Read the model definition and answer for the solid it produces. Units are mm, in the model's axes. Face numbers are marked on the shaded views. A direction names the side the tool comes from. Give positions to 0.01 mm unless a question says otherwise; leave off trailing zeros. Write each loop counter-clockwise with the first axis right and the second up, starting at its lowest first coordinate (ties: lowest second). Pieces come first, ordered by that corner, then holes. Notation, with made-up numbers: M 83.5,-4 L 106.5,-4 A3 ccw 106.5,0 Z; hole C 29,26.25 d6. An arc over 180 degrees is marked long. Put each result on its own line as item: value.
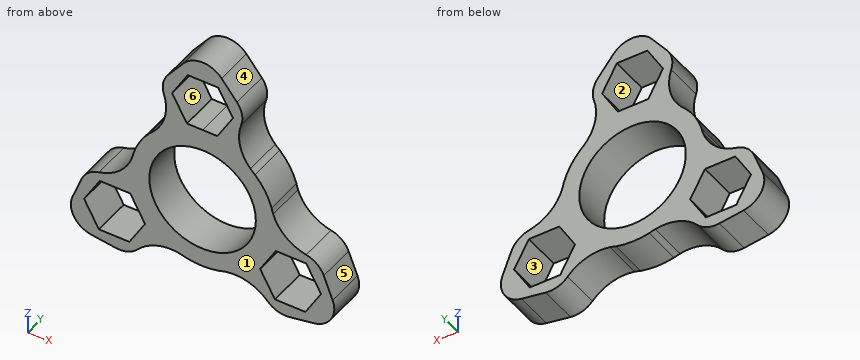
from build123d import *

# Parameters (mm, degrees)
F0_R     = 10.9
F1_DEPTH = 8
F2_R     = 5


with BuildPart() as f1:
    # F0 (on Front) → F1 (new body)
    with BuildSketch(Plane.XZ):
        with BuildLine():
            ThreePointArc((-4.6474292299, -13.9936443391), (-12.7697106566, -7.372595885), (-14.4425661041, 2.9720303942))
            ThreePointArc((-14.4425661041, 2.9720303942), (-17.9890829323, -1.7394577094), (-23.6744608764, -3.305465179))
            Line((-23.6744608764, -3.305465179), (-26.6141080798, -10.8626586404))
            ThreePointArc((-26.6141080798, -10.8626586404), (-26.2843656104, -15.1752855606), (-22.7143923751, -17.617164376))
            Line((-22.7143923751, -17.617164376), (-14.6998472546, -18.8499519504))
            ThreePointArc((-14.6998472546, -18.8499519504), (-10.5009560313, -14.7092739554), (-4.6474292299, -13.9936443391))
        make_face()
        Polygon((-21.2154018643, -15.7464514283), (-24.2445278885, -10.2962775292), (-21.039101849, -4.9478904915), (-14.8045497853, -5.0496773528), (-11.7754237611, -10.4998512519), (-14.9808498006, -15.8482382896), align=None, mode=Mode.SUBTRACT)
        with BuildLine():
            ThreePointArc((9.7951368743, 11.0216139449), (5.2395070905, 13.7828968575), (0, 14.7451917701))
            ThreePointArc((0, 14.7451917701), (-5.2395070905, 13.7828968575), (-9.7951368743, 11.0216139449))
            ThreePointArc((-9.7951368743, 11.0216139449), (-10.2405850834, 10.5580719376), (-10.7175072848, 10.1269797045))
            ThreePointArc((-10.7175072848, 10.1269797045), (-12.7697106566, 7.372595885), (-14.1289753301, 4.2181437217))
            ThreePointArc((-14.1289753301, 4.2181437217), (-14.2638510546, 3.5895708631), (-14.4425661041, 2.9720303942))
            ThreePointArc((-14.4425661041, 2.9720303942), (-12.7697106566, -7.372595885), (-4.6474292299, -13.9936443391))
            ThreePointArc((-4.6474292299, -13.9936443391), (-4.0232659712, -14.1476428006), (-3.4114680453, -14.3451234262))
            ThreePointArc((-3.4114680453, -14.3451234262), (0, -14.7451917701), (3.4114680453, -14.3451234262))
            ThreePointArc((3.4114680453, -14.3451234262), (4.0232659712, -14.1476428006), (4.6474292299, -13.9936443391))
            ThreePointArc((4.6474292299, -13.9936443391), (11.9571718138, -8.6282514191), (14.7451917701, 0))
            ThreePointArc((14.7451917701, 0), (14.6693402577, 1.4936990123), (14.4425661041, 2.9720303942))
            ThreePointArc((14.4425661041, 2.9720303942), (14.2638510546, 3.5895708631), (14.1289753301, 4.2181437217))
            ThreePointArc((14.1289753301, 4.2181437217), (12.7697106566, 7.372595885), (10.7175072848, 10.1269797045))
            ThreePointArc((10.7175072848, 10.1269797045), (10.2405850834, 10.5580719376), (9.7951368743, 11.0216139449))
        make_face()
        Circle(F0_R, mode=Mode.SUBTRACT)
        with BuildLine():
            ThreePointArc((23.6744608764, -3.305465179), (17.9890829323, -1.7394577094), (14.4425661041, 2.9720303942))
            ThreePointArc((14.4425661041, 2.9720303942), (14.6693402577, 1.4936990123), (14.7451917701, 0))
            ThreePointArc((14.7451917701, 0), (11.9571718138, -8.6282514191), (4.6474292299, -13.9936443391))
            ThreePointArc((4.6474292299, -13.9936443391), (10.5009560313, -14.7092739554), (14.6998472546, -18.8499519504))
            Line((14.6998472546, -18.8499519504), (22.7143923751, -17.617164376))
            ThreePointArc((22.7143923751, -17.617164376), (26.2843656104, -15.1752855606), (26.6141080798, -10.8626586404))
            Line((26.6141080798, -10.8626586404), (23.6744608764, -3.305465179))
        make_face()
        Polygon((24.2445278885, -10.4998512519), (21.039101849, -15.8482382896), (14.8045497853, -15.7464514283), (11.7754237611, -10.2962775292), (14.9808498006, -4.9478904915), (21.2154018643, -5.0496773528), align=None, mode=Mode.SUBTRACT)
        with BuildLine():
            ThreePointArc((-9.7951368743, 11.0216139449), (-5.2395070905, 13.7828968575), (0, 14.7451917701))
            ThreePointArc((0, 14.7451917701), (5.2395070905, 13.7828968575), (9.7951368743, 11.0216139449))
            ThreePointArc((9.7951368743, 11.0216139449), (7.488126901, 16.4487316648), (8.9746136218, 22.1554171294))
            Line((8.9746136218, 22.1554171294), (3.8997157047, 28.4798230164))
            ThreePointArc((3.8997157047, 28.4798230164), (0, 30.3505711213), (-3.8997157047, 28.4798230164))
            Line((-3.8997157047, 28.4798230164), (-8.9746136218, 22.1554171294))
            ThreePointArc((-8.9746136218, 22.1554171294), (-7.488126901, 16.4487316648), (-9.7951368743, 11.0216139449))
        make_face()
        Polygon((3.0291260242, 15.3459548821), (0, 15.3954091536), (-3.2054260395, 15.4477417434), (-6.2345520637, 20.8979156424), (-3.0291260242, 26.2463026801), (3.2054260395, 26.1445158188), (6.2345520637, 20.6943419198), align=None, mode=Mode.SUBTRACT)
    extrude(amount=F1_DEPTH)

    # F2
    f2_edges = [f1.edges().sort_by_distance(p)[0] for p in [
        (-23.674461, -4, -3.305465),
        (-14.699847, -4, -18.849952),
        (14.699847, -4, -18.849952),
        (23.674461, -4, -3.305465),
        (8.974614, -4, 22.155417),
        (-8.974614, -4, 22.155417),
    ]]
    fillet(f2_edges, radius=F2_R)


solid = f1.part
(1) Which of the six approach directions +Z, -Z, +X, -X, +Y, -Y give full straight-line access (tool end or side, diameter ignored) to the marked faces 5 and 6?
Result:
face 5: +Z, +X, +Y, -Y
face 6: +Y, -Y
(2) Section B-B on z = 0 is taken. Determine the outline of the cut face in (x, y).
Result:
outline: M -16.08,-8 L -10.9,-8 L -10.9,0 L -16.08,0 Z; M 10.9,-8 L 16.08,-8 L 16.08,0 L 10.9,0 Z
(3) Straight lines are drawn through the part: line 1 along Z through (x, y) = (-0.5, -7); line 2 along X through (y, z) = (-5.75, -15.5); line 3 along Z through (x, y) = (1, -0.5). For each, find the intervals that lie inside material, in ascending order. Write a range as from..to.
Result:
line 1: z = -14.74..-10.89, 10.89..15.4, 26.21..30.33
line 2: x = -26.08..-21.35, -14.77..-11.84, 11.84..14.67, 21.25..26.08
line 3: z = -14.71..-10.85, 10.85..15.38, 26.18..30.25
(4) Section C-C on y = -2.5 is taken. Give the number of separate pieces and of enclosed holes in the cut face, and give its area (3 significant figures).
Result:
separate pieces: 1
enclosed holes: 4
area: 663 mm²
(5) Section A-A on x = -19 is taken. Determine the outline of the cut face in (y, z), and give its area (3 significant figures).
Result:
outline: M -8,-18.19 L 0,-18.19 L 0,-15.78 L -8,-15.78 Z; M -8,-4.98 L 0,-4.98 L 0,-2.34 L -8,-2.34 Z
area: 40.4 mm²
(6) Given pin 1 Ø8 at (x, z) = (1.5, -4.5) entering from -Y; pin 2 Ø3 at (y, z) = (-4, 17.5) entering from +X, each flat-ended and moving along its own axis, determine where each tip first touches the part or whether it passes through.
Result:
pin 1: passes through
pin 2: stops at x = 7.66
(7) For a pull along Z with two mould halves and no side action, classify the marked faces 1, 2, 3 and 4 as +Z half, -Z half, draft (parallel to the pull), parting line (faces both ways), or undercut.
Result:
face 1: draft
face 2: undercut
face 3: undercut
face 4: +Z half
